```python
from build123d import *

# Parameters (mm, degrees)
SKETCH1_R               = 3.175
BOSS_EXTRUDE1_DEPTH     = 5.08
CUT_EXTRUDE2_DEPTH      = 5.715
CUT_EXTRUDE3_DEPTH      = 120.302535254
CUT_EXTRUDE3_DEPTH_BACK = 120.302535254
SKETCH4_R               = 0.396875
CUT_EXTRUDE8_DEPTH      = 1.905


with BuildPart() as part:
    # Sketch1 → Boss-Extrude1 (new, symmetric)
    with BuildSketch(Plane(origin=(0, 0, 0), x_dir=(1, 0, 0), z_dir=(0, 1, 0))):
        with BuildLine():
            ThreePointArc((-12.7, 101.6), (-17.514407624, 57.062136043), (-31.735205033, 14.581919851))
            ThreePointArc((-31.735205033, 14.581919851), (0, -34.925), (31.735205033, 14.581919851))
            ThreePointArc((31.735205033, 14.581919851), (17.514407624, 57.062136043), (12.7, 101.6))
            ThreePointArc((12.7, 101.6), (0, 114.3), (-12.7, 101.6))
        make_face()
        with Locations(Location((0, 0, 0), (0, 0, 270))):
            Circle(SKETCH1_R, mode=Mode.SUBTRACT)
    extrude(amount=BOSS_EXTRUDE1_DEPTH, both=True)

    # Sketch2 → Cut-Extrude2 (cut, symmetric)
    with BuildSketch(Plane(origin=(0, 0, 0), x_dir=(1, 0, 0), z_dir=(0, 1, 0))):
        with BuildLine():
            ThreePointArc((-2.500603456, 105.207450456), (-2.42672892, 106.304643007), (-2.500603456, 107.401835557))
            ThreePointArc((-2.500603456, 107.401835557), (-3.18246494, 108.814648011), (-3.123385981, 110.382284382))
            ThreePointArc((-3.123385981, 110.382284382), (-2.80162, 112.654643007), (-3.123385981, 114.927001632))
            ThreePointArc((-3.123385981, 114.927001632), (-3.18246494, 116.494638003), (-2.500603456, 117.907450456))
            ThreePointArc((-2.500603456, 117.907450456), (-2.42672892, 119.004643007), (-2.500603456, 120.101835557))
            ThreePointArc((-2.500603456, 120.101835557), (-3.18246494, 121.514648011), (-3.123385981, 123.082284382))
            ThreePointArc((-3.123385981, 123.082284382), (-2.80162, 125.354643007), (-3.123385981, 127.627001632))
            ThreePointArc((-3.123385981, 127.627001632), (-3.18246494, 129.194638003), (-2.500603456, 130.607450456))
            ThreePointArc((-2.500603456, 130.607450456), (-2.451700025, 132.343502027), (-2.77019509, 134.050788615))
            ThreePointArc((-2.77019509, 134.050788615), (0, 137.771179007), (2.77019509, 134.050788615))
            ThreePointArc((2.77019509, 134.050788615), (2.451700025, 132.343502027), (2.500603456, 130.607450456))
            ThreePointArc((2.500603456, 130.607450456), (3.18246494, 129.194638003), (3.123385981, 127.627001632))
            ThreePointArc((3.123385981, 127.627001632), (2.80162, 125.354643007), (3.123385981, 123.082284382))
            ThreePointArc((3.123385981, 123.082284382), (3.18246494, 121.514648011), (2.500603456, 120.101835557))
            ThreePointArc((2.500603456, 120.101835557), (2.42672892, 119.004643007), (2.500603456, 117.907450456))
            ThreePointArc((2.500603456, 117.907450456), (3.18246494, 116.494638003), (3.123385981, 114.927001632))
            ThreePointArc((3.123385981, 114.927001632), (2.80162, 112.654643007), (3.123385981, 110.382284382))
            ThreePointArc((3.123385981, 110.382284382), (3.18246494, 108.814648011), (2.500603456, 107.401835557))
            ThreePointArc((2.500603456, 107.401835557), (2.42672892, 106.304643007), (2.500603456, 105.207450456))
            ThreePointArc((2.500603456, 105.207450456), (3.18246494, 103.794638003), (3.123385981, 102.227001632))
            ThreePointArc((3.123385981, 102.227001632), (2.80162, 99.954643007), (3.123385981, 97.682284382))
            ThreePointArc((3.123385981, 97.682284382), (3.18246494, 96.114648011), (2.500603456, 94.701835557))
            ThreePointArc((2.500603456, 94.701835557), (2.42672892, 93.604643007), (2.500603456, 92.507450456))
            ThreePointArc((2.500603456, 92.507450456), (3.18246494, 91.094638003), (3.123385981, 89.527001632))
            ThreePointArc((3.123385981, 89.527001632), (2.80162, 87.254643007), (3.123385981, 84.982284382))
            ThreePointArc((3.123385981, 84.982284382), (0, 80.828443007), (-3.123385981, 84.982284382))
            ThreePointArc((-3.123385981, 84.982284382), (-2.80162, 87.254643007), (-3.123385981, 89.527001632))
            ThreePointArc((-3.123385981, 89.527001632), (-3.18246494, 91.094638003), (-2.500603456, 92.507450456))
            ThreePointArc((-2.500603456, 92.507450456), (-2.42672892, 93.604643007), (-2.500603456, 94.701835557))
            ThreePointArc((-2.500603456, 94.701835557), (-3.18246494, 96.114648011), (-3.123385981, 97.682284382))
            ThreePointArc((-3.123385981, 97.682284382), (-2.80162, 99.954643007), (-3.123385981, 102.227001632))
            ThreePointArc((-3.123385981, 102.227001632), (-3.18246494, 103.794638003), (-2.500603456, 105.207450456))
        make_face()
    extrude(amount=CUT_EXTRUDE2_DEPTH, both=True, mode=Mode.SUBTRACT)

    # Sketch4 → Cut-Extrude3 (cut, two sides: drawn at the far end of the back side and taken through both)
    with BuildSketch(Plane(origin=(0, 0, 0), x_dir=(0, 0, -1), z_dir=(1, 0, 0)).offset(-CUT_EXTRUDE3_DEPTH_BACK)):
        with Locations((87.254643007, 0)):
            Circle(SKETCH4_R)
        with Locations((99.954643007, 0)):
            Circle(SKETCH4_R)
    extrude(amount=CUT_EXTRUDE3_DEPTH + CUT_EXTRUDE3_DEPTH_BACK, mode=Mode.SUBTRACT)

    # Sketch11 → Cut-Extrude8 (cut)
    with BuildSketch(Plane(origin=(0, 5.08, 0), x_dir=(1, 0, 0), z_dir=(0, 1, 0))):
        with BuildLine():
            Line((-34.908444977, 1.075218257), (-31.734949979, 104.107114149))
            ThreePointArc((-31.734949979, 104.107114149), (0, 71.379643007), (31.734949979, 104.107114149))
            Line((31.734949979, 104.107114149), (34.908444977, 1.075218257))
            ThreePointArc((34.908444977, 1.075218257), (0, -34.925), (-34.908444977, 1.075218257))
        make_face()
    cut_extrude8 = extrude(amount=-CUT_EXTRUDE8_DEPTH, mode=Mode.SUBTRACT)

    # Mirror1: Cut-Extrude8 across plane
    add(cut_extrude8.mirror(Plane.ZX), mode=Mode.SUBTRACT)


solid = part.part
```
CAD build for the part. Positions are in the model's coordinates, mm. A direction names the side the tool comes from. Give positions to 0.01 mm unless a question says otherwise; leave off trailing zeros. Loops run counter-clockwise (first coordinate to the right, second up) from the corner with the lowest first, then second, coordinate; pieces in that order, holes last. Notation, with made-up numbers: (87, 17) - (96, 17) arc R11 ccw to (96, 35) - close; hole circle Ø9 at (37, -22.75). An arc over 180 degrees is marked (long way). Put each result on its own line as item: value.
Q1. Slice it at A-A (x = 0). Give the cut face in (y, z) (3 decimals), plus the area to 3 significant figures.
Filled in:
outline: (-5.08, -80.828) - (5.08, -80.828) - (5.08, -71.38) - (3.175, -71.38) - (3.175, -3.175) - (-3.175, -3.175) - (-3.175, -71.38) - (-5.08, -71.38) - close; (-3.175, 3.175) - (3.175, 3.175) - (3.175, 34.925) - (-3.175, 34.925) - close
area: 731 mm²
Q2. Flat gauge pins, fed straight in: pin 1 (1 mm diameter, centred on x = 2.5, z = -34, fed in from +Y) (3 decimals); pin 2 (5 mm diameter, centred on y = 3.5, z = -65.5, fed in from +X); pin 3 (4 mm diameter, centred on x = 0, z = 0, fed in from -Y); pin 4 (10 mm diameter, centred on x = 15, z = -54.5, fed in from -Y) (3 decimals). Where does each tip first touch, or does it go through?
Filled in:
pin 1: stops at y = 3.175
pin 2: stops at x = 16.3
pin 3: passes through
pin 4: stops at y = -3.175
Q3. Probe line 1 along Z through (x, y) = (10, 0); line 2 along Z through (x, y) = (-10.5, 0); line 3 along Y through (x, z) = (-19, -20.5) (3 decimals). List the from-to ranges inside material, lowest first.
Filled in:
line 1: z = -109.43 to -100.35, -99.56 to -87.65, -86.86 to 33.46
line 2: z = -108.74 to -100.35, -99.56 to -87.65, -86.86 to 33.31
line 3: y = -3.175 to 3.175
Q4. Mould opens along Z. For faces 4 (the face through (-0.21, -4.14, -71.38)), 5 (the face through (0.08, 0.07, -80.83)), 6 (the face through (15.723, 0.071, -66.234)), 7 (the face through (3, 5.08, -93)) say: pulls with the +Z half, pulls with the -Z half, needs draft (parallel to the pull), parting line crosses it, or undercut.
Filled in:
face 4: pulls with the +Z half
face 5: undercut
face 6: pulls with the -Z half
face 7: needs draft
Q5. Tool access for faces 1 (the face through (3.178, 0.071, -91.116)), 2 (the face through (-0.21, 4.14, -71.38)), 3 (the face through (-15.513, 0.071, -67.473)): list every direction of +Z, -Z, +X, -X, +Y, -Y with a clear straight run to the whole face (end or side of a thin tool).
Filled in:
face 1: +Y, -Y
face 2: +Z, +Y
face 3: -Z, -X, +Y, -Y
Q6. Slice it at C-C (x = 28). Give the cut face in (y, z) (3 decimals), plus the area to 3 significant figures.
Filled in:
outline: (-3.175, -23.22) - (3.175, -23.22) - (3.175, 20.875) - (-3.175, 20.875) - close
area: 280 mm²
Q7. Slice it at B-B (z = -43.5). Give the cut face in (x, y) (3 decimals), plus the area to 3 significant figures.
Filled in:
outline: (-20.962, -3.175) - (20.962, -3.175) - (20.962, 3.175) - (-20.962, 3.175) - close
area: 266 mm²
